from build123d import *

# Parameters (mm, degrees)
PRISM001_DEPTH    = 3.5
CYLINDER006_R     = 2.95
CYLINDER006_DEPTH = 25
CYLINDER005_R     = 10
CYLINDER005_DEPTH = 13
CYLINDER007_R     = 2.85
CYLINDER007_DEPTH = 25
BOX002_W          = 62
BOX002_H          = 8
BOX002_DEPTH      = 22


with BuildPart() as prisma001:
    # Prism001 → Prism001 (new body)
    with BuildSketch(Plane(origin=(0, 8, 9), x_dir=(1, 0, 0), z_dir=(0, -1, 0))):
        Polygon((3.5, 0), (1.75, 3.031089), (-1.75, 3.031089), (-3.5, 0), (-1.75, -3.031089), (1.75, -3.031089), align=None)
    extrude(amount=PRISM001_DEPTH)


with BuildPart() as cilindro006:
    # Cylinder006 → Cylinder006 (new body)
    with BuildSketch(Plane.XY.offset(-7)):
        Circle(CYLINDER006_R)
    extrude(amount=CYLINDER006_DEPTH)


with BuildPart() as cut006:
    # Cylinder005 → Cylinder005 (new body)
    with BuildSketch(Plane.XY):
        Circle(CYLINDER005_R)
    extrude(amount=CYLINDER005_DEPTH)

    # Cut005: cut Cilindro006
    add(cilindro006.part, mode=Mode.SUBTRACT)

    # Cut006: cut Prisma001
    add(prisma001.part, mode=Mode.SUBTRACT)


with BuildPart() as cilindro007:
    # Cylinder007 → Cylinder007 (new body)
    with BuildSketch(Plane.XY.offset(-7)):
        Circle(CYLINDER007_R)
    extrude(amount=CYLINDER007_DEPTH)


with BuildPart() as fusion:
    # Box002 → Box002 (new body)
    with BuildSketch(Plane(origin=(-31, 11, 0), x_dir=(1, 0, 0), z_dir=(0, -1, 0))):
        with Locations((31, 4)):
            Rectangle(BOX002_W, BOX002_H)
    extrude(amount=BOX002_DEPTH)

    # Cut: cut Cilindro007
    add(cilindro007.part, mode=Mode.SUBTRACT)

    # Fusion: union Cut006
    add(cut006.part)


solid = fusion.part
Source: CAD feature listing. Evaluate the final solid. Frame: model axes, mm. A direction names the side the tool comes from. Give positions to 0.01 mm unless a question says otherwise; leave off trailing zeros. Loops run counter-clockwise (first coordinate to the right, second up) from the corner with the lowest first, then second, coordinate; pieces in that order, holes last. Notation, with made-up numbers: (45.5, -32.5) -> (64.5, -32.5) arc R18 cw to (64.5, -19.5) -> close; hole circle Ø8 at (-29.5, -21.5). An arc over 180 degrees is marked (long way). Use a Markdown table: item, result. Add a question column.
1) Section query A-A, the plane x = 0. Return the cut outline in (y, z).
2) First-contact query: pin 1 (3 mm diameter, centred on x = -0.5, z = 10.5, fed in from -Y); pin 2 (3 mm diameter, centred on x = -11.5, y = 1.5, fed in from +Z); pin 3 (11 mm diameter, centred on x = 14.5, y = 0, fed in from +Z); pin 4 (4.5 mm diameter, centred on x = -1.5, z = 10.5, fed in from +Y). Flat tips, straight axial feed; report the tip coordinate or a pass-through.
3) Section query D-D, the plane y = 9. Return the cut outline in (x, z), then the cut area to 3 significant figures.
4) Section query C-C, the plane z = 2. Return the cut outline in (x, y).
5) Reachability of faces 4 (the face through (0, -5, 0)), 5 (the face through (-2.947, 0.13, 10.465)), 6 (the face through (-2.61, 6.27, 10.54)) from +Z, -Z, +X, -X, +Y, -Y: full face, straight path, thin tool, end or side. Return the list, or none.
6) Pull-direction query (Z, two-part tool) for faces 1 (the face through (0, 11, 4)), 2 (the face through (-7.3, 7.5, 8)), 3 (the face through (0, 8, 10)); classes: +Z half, -Z half, draft (parallel to the pull), parting line (faces both ways), or undercut.
7) Line query: line 1 along Y through (x, z) = (0, 10); line 2 along Y through (x, z) = (0, 6.25); line 3 along X through (y, z) = (0, 12.25). Output: solid intervals per line, ascending. Write a range as [from, to].
8) Section query B-B, the plane y = 0. Return the cut outline in (x, z).
Numbers:
| question | item | result |
|---|---|---|
| 1 | outline | (-11, 0) -> (-2.85, 0) -> (-2.85, 8) -> (-2.95, 8) -> (-2.95, 13) -> (-10, 13) -> (-10, 8) -> (-11, 8) -> close; (2.85, 0) -> (11, 0) -> (11, 8) -> (10, 8) -> (10, 13) -> (2.95, 13) -> (2.95, 8) -> (2.85, 8) -> close; hole (4.5, 8) -> (8, 8) -> (8, 12.03) -> (4.5, 12.03) -> close |
| 2 | pin 1 | stops at y = -10 |
| 2 | pin 2 | stops at z = 8 |
| 2 | pin 3 | stops at z = 13 |
| 2 | pin 4 | stops at y = 10 |
| 3 | outline | (-31, 0) -> (31, 0) -> (31, 8) -> (4.36, 8) -> (4.36, 13) -> (-4.36, 13) -> (-4.36, 8) -> (-31, 8) -> close |
| 3 | area | 540 mm2 |
| 4 | outline | (-31, -11) -> (31, -11) -> (31, 11) -> (-31, 11) -> close; hole circle Ø5.7 at (0, 0) |
| 5 | face 4 | -Z, +X, -X, +Y, -Y |
| 5 | face 5 | +Z |
| 5 | face 6 | none |
| 6 | face 1 | draft |
| 6 | face 2 | +Z half |
| 6 | face 3 | undercut |
| 7 | line 1 | y = [-10, -2.95], [2.95, 4.5], [8, 10] |
| 7 | line 2 | y = [-11, -2.85], [2.85, 11] |
| 7 | line 3 | x = [-10, -2.95], [2.95, 10] |
| 8 | outline | (-31, 0) -> (-2.85, 0) -> (-2.85, 8) -> (-2.95, 8) -> (-2.95, 13) -> (-10, 13) -> (-10, 8) -> (-31, 8) -> close; (2.85, 0) -> (31, 0) -> (31, 8) -> (10, 8) -> (10, 13) -> (2.95, 13) -> (2.95, 8) -> (2.85, 8) -> close |
